Build history of the part. All positions in model axes, mm. A direction names the side the tool comes from. Coordinates: 2 decimals unless noted, no trailing zeros. Loops run counter-clockwise (first coordinate to the right, second up) from the corner with the lowest first, then second, coordinate; pieces in that order, holes last.
(1) Slice it at D-D (x = -3.75). Give the cut face in (y, z).
(2) Slice it at C-C (z = -1.45). Give the cut face in (x, y), and give its area (3 significant figures).
(3) Flat gauge pin, fed straight in: P1, Ø6, axis at x = 0, y = -13, coming from the +Z side. Where does the tip first touch, or does it go through?
(4) Slice it at B-B (y = 13). Give the cut face in (x, z), and give its area (3 significant figures).
(5) Wall check: L1, parallel to Y at x = 0, z = -1.75; L2, parallel to Y at x = -1.5, z = 0.4; L3, parallel to X at y = 12.5, z = -2.65. Give the ranges that are in metal, low to high.
(6) Tool access for faces 1 (the face through (0.105, -8.733, 1.986)), 2 (the face through (0, -16, 3)): list every direction of +Z, -Z, +X, -X, +Y, -Y with a clear straight run to the whole face (end or side of a thin tool).
(7) Slice it at A-A (x = 0). Give the cut face in (y, z).
from build123d import *

# Parameters (mm, degrees)
SKETCH_1_W             = 15
SKETCH_1_H             = 38
SKETCH_1_R             = 2.25
EXTRUDE_1_DEPTH        = 3
FILLET_1_R             = 0.5
CUT_EXTRUDE_1_DEPTH    = 7.5
PATTERN_LINEAR_1_COUNT = 4
PATTERN_LINEAR_1_PITCH = 5


with BuildPart() as part:
    # 草图1 → 凸台-拉伸1 (new, symmetric)
    with BuildSketch(Plane.XY):
        Rectangle(SKETCH_1_W, SKETCH_1_H)
        with Locations((0, 13)):
            Circle(SKETCH_1_R, mode=Mode.SUBTRACT)
        with Locations((0, -13)):
            Circle(SKETCH_1_R, mode=Mode.SUBTRACT)
    extrude(amount=EXTRUDE_1_DEPTH, both=True)

    # 圆角1
    fillet_1_edges = [part.edges().sort_by_distance(p)[0] for p in [
        (-7.5, 0, 3),
        (0, -19, 3),
        (7.5, 0, 3),
        (0, -19, -3),
        (-7.5, 0, -3),
        (0, 19, -3),
        (7.5, 0, -3),
        (7.5, -19, 0),
        (-7.5, -19, 0),
        (-7.5, 19, 0),
        (7.5, 19, 0),
        (0, 19, 3),
    ]]
    fillet(fillet_1_edges, radius=FILLET_1_R)

    # 草图2 → 切除-拉伸1 (cut, symmetric)
    with BuildSketch(Plane(origin=(0, 0, 0), x_dir=(0, 0, -1), z_dir=(1, 0, 0))):
        Polygon((-3, 10), (-1, 7.5), (-3, 5), align=None)
    cut_extrude_1 = extrude(amount=CUT_EXTRUDE_1_DEPTH, both=True, mode=Mode.SUBTRACT)

    # 阵列(线性)1: 切除-拉伸1 ×4
    with Locations(*[(0, -i * PATTERN_LINEAR_1_PITCH, 0) for i in range(1, PATTERN_LINEAR_1_COUNT)]):
        add(cut_extrude_1, mode=Mode.SUBTRACT)


solid = part.part
Response values:
1. outline: (-19, -2.5) arc R0.5 ccw to (-18.5, -3) - (18.5, -3) arc R0.5 ccw to (19, -2.5) - (19, 2.5) arc R0.5 ccw to (18.5, 3) - (10, 3) - (7.5, 1) - (5, 3) - (2.5, 1) - (0, 3) - (-2.5, 1) - (-5, 3) - (-7.5, 1) - (-10, 3) - (-18.5, 3) arc R0.5 ccw to (-19, 2.5) - close
2. outline: (-7.5, -18.5) arc R0.5 ccw to (-7, -19) - (7, -19) arc R0.5 ccw to (7.5, -18.5) - (7.5, 18.5) arc R0.5 ccw to (7, 19) - (-7, 19) arc R0.5 ccw to (-7.5, 18.5) - close; hole circle Ø4.5 at (0, -13); hole circle Ø4.5 at (0, 13)
2. area: 538 mm2
3. P1: stops at z = 3
4. outline: (-7.5, -2.5) arc R0.5 ccw to (-7, -3) - (-2.25, -3) - (-2.25, 3) - (-7, 3) arc R0.5 ccw to (-7.5, 2.5) - close; (2.25, -3) - (7, -3) arc R0.5 ccw to (7.5, -2.5) - (7.5, 2.5) arc R0.5 ccw to (7, 3) - (2.25, 3) - close
4. area: 62.8 mm2
5. L1: y = -19 to -15.25, -10.75 to 10.75, 15.25 to 19
5. L2: y = -19 to -14.68, -11.32 to 11.32, 14.68 to 19
5. L3: x = -7.48 to -2.19, 2.19 to 7.48
6. face 1: +Z, +X, -X
6. face 2: +Z, +X, -X, +Y, -Y
7. outline: (-19, -2.5) arc R0.5 ccw to (-18.5, -3) - (-15.25, -3) - (-15.25, 3) - (-18.5, 3) arc R0.5 ccw to (-19, 2.5) - close; (-10.75, -3) - (10.75, -3) - (10.75, 3) - (10, 3) - (7.5, 1) - (5, 3) - (2.5, 1) - (0, 3) - (-2.5, 1) - (-5, 3) - (-7.5, 1) - (-10, 3) - (-10.75, 3) - close; (15.25, -3) - (18.5, -3) arc R0.5 ccw to (19, -2.5) - (19, 2.5) arc R0.5 ccw to (18.5, 3) - (15.25, 3) - close
